For this review, take the finished solid that the model builds, in its own axes (mm). Coordinates: 2 decimals unless noted, no trailing zeros. Loops run counter-clockwise (first coordinate to the right, second up) from the corner with the lowest first, then second, coordinate; pieces in that order, holes last.
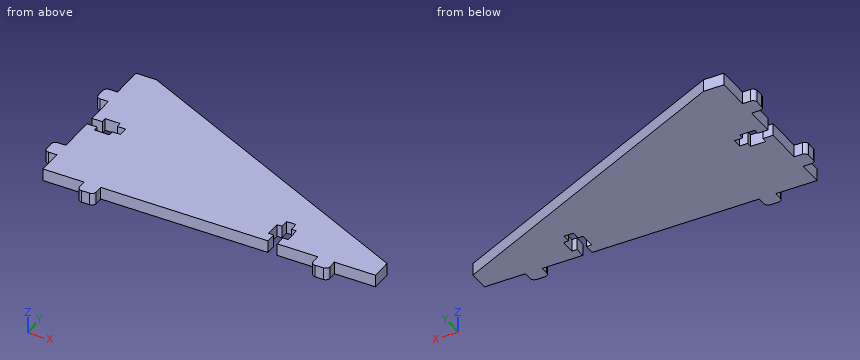
Autodesk Inventor part; units mm, degrees
ref_plane "YZ Plane" through (0, 0, 0) normal (1, 0, 0) x (0, 1, 0)
ref_plane "XZ Plane" through (0, 0, 0) normal (0, 1, 0) x (-1, 0, 0)
ref_plane "XY Plane" through (0, 0, 0) normal (0, 0, 1) x (1, 0, 0)
sketch "Sketch1" plane through (0, 0, 0) normal (0, 0, 1) x (1, 0, 0)
  line L0 (0, 81) -> (0, 0)
  line L1 (0, 0) -> (161.5, 0)
  line L2 (161.5, 0) -> (161.5, 10)
  line L3 (161.5, 10) -> (10, 81)
  line L4 (10, 81) -> (0, 81)
  dimension "d0" = 161.5
  dimension "d1" = 81
  dimension "d2" = 10
  dimension "d3" = 10
extrude "Extrusion1" add sketch "Sketch1" along normal blind 6
sketch "Sketch2" plane through (0, 0, 6) normal (0, 0, 1) x (1, 0, 0)
  line L0 (0, 81) -> (0, 0)
  line L1 (0, 0) -> (161.5, 0)
  line L2 (161.5, 0) -> (161.5, 10)
  line L3 (16.3, 42.75) -> (16.3, 38.25)
  line L4 (0, 38.25) -> (0, 42.75)
  line L5 (5, 45.25) -> (12.3, 45.25)
  line L6 (12.3, 35.75) -> (5, 35.75)
  line L7 (0, 42.75) -> (5, 42.75)
  line L8 (12.3, 42.75) -> (16.3, 42.75)
  line L9 (16.3, 38.25) -> (12.3, 38.25)
  line L10 (5, 38.25) -> (0, 38.25)
  line L11 (5, 35.75) -> (5, 38.25)
  line L12 (5, 42.75) -> (5, 45.25)
  line L13 (12.3, 45.25) -> (12.3, 42.75)
  line L14 (12.3, 38.25) -> (12.3, 35.75)
  line L15 (109.25, 16.3) -> (113.75, 16.3)
  line L16 (113.75, 0) -> (109.25, 0)
  line L17 (116.25, 12.3) -> (116.25, 5)
  line L18 (106.75, 5) -> (106.75, 12.3)
  line L19 (106.75, 12.3) -> (109.25, 12.3)
  line L20 (113.75, 12.3) -> (116.25, 12.3)
  line L21 (116.25, 5) -> (113.75, 5)
  line L22 (109.25, 5) -> (106.75, 5)
  line L23 (109.25, 0) -> (109.25, 5)
  line L24 (109.25, 12.3) -> (109.25, 16.3)
  line L25 (113.75, 16.3) -> (113.75, 12.3)
  line L26 (113.75, 5) -> (113.75, 0)
  point P0 (16.3, 40.5)
  point P1 (0, 40.5)
  point P2 (111.5, 16.3)
  dimension "d6" = 4.5
  dimension "d7" = 2.5
  dimension "d8" = 2.5
  dimension "d9" = 5
  dimension "d10" = 7.3
  dimension "d11" = 4
  dimension "d12" = 4.5
  dimension "d13" = 5
  dimension "d14" = 7.3
  dimension "d15" = 4
  dimension "d16" = 2.5
  dimension "d17" = 2.5
  dimension "d18" = 50
extrude "Extrusion2" cut sketch "Sketch2" against normal blind 6
sketch "Sketch3" plane through (0, 0, 6) normal (0, 0, 1) x (1, 0, 0)
  line L0 (0, 38.25) -> (0, 0)
  line L1 (0, 0) -> (109.25, 0)
  line L2 (113.75, 0) -> (161.5, 0)
  line L3 (10, 81) -> (0, 81)
  line L4 (0, 81) -> (0, 42.75)
  line L5 (0, 65) -> (-4, 65)
  line L6 (-6, 63) -> (-6, 59)
  line L7 (-4, 57) -> (0, 57)
  line L8 (0, 57) -> (0, 65)
  line L9 (0, 20) -> (-4, 20)
  line L10 (-6, 18) -> (-6, 14)
  line L11 (-4, 12) -> (0, 12)
  line L12 (0, 12) -> (0, 20)
  line L13 (20, 0) -> (28, 0)
  line L14 (28, 0) -> (28, -4)
  line L15 (26, -6) -> (22, -6)
  line L16 (20, -4) -> (20, 0)
  line L17 (133.5, 0) -> (141.5, 0)
  line L18 (141.5, 0) -> (141.5, -4)
  line L19 (139.5, -6) -> (135.5, -6)
  line L20 (133.5, -4) -> (133.5, 0)
  arc A0 (-4, 65) -> (-6, 63) centre (-4, 63) ccw
  arc A1 (-6, 59) -> (-4, 57) centre (-4, 59) ccw
  arc A2 (-4, 20) -> (-6, 18) centre (-4, 18) ccw
  arc A3 (-6, 14) -> (-4, 12) centre (-4, 14) ccw
  arc A4 (20, -4) -> (22, -6) centre (22, -4) ccw
  arc A5 (26, -6) -> (28, -4) centre (26, -4) ccw
  arc A6 (133.5, -4) -> (135.5, -6) centre (135.5, -4) ccw
  arc A7 (139.5, -6) -> (141.5, -4) centre (139.5, -4) ccw
  dimension "d21" = 2
  dimension "d22" = 8
  dimension "d23" = 8
  dimension "d24" = 8
  dimension "d25" = 8
  dimension "d26" = 6
  dimension "d27" = 6
  dimension "d28" = 12
  dimension "d29" = 16
  dimension "d30" = 20
  dimension "d31" = 20
extrude "Extrusion3" add sketch "Sketch3" against normal blind 6
properties part number "wiring_brace"
Q1. Consider section A-A (x = 67.5). State the section outline as (y, z) points.
Q2. Consider section B-B (y = 28). State the section outline as (x, z) points.
Q3. Wall thickness on probe 1 along X at (y, z) = (2.5, 5.15); probe 2 along X at (y, z) = (9, 3.35); probe 3 along Y at (x, z) = (153, 4.5): over which ranges is each line inside the solid? List them lowest first.
Q4. For pin 1 Ø1.5 at (y, z) = (27.5, 3.5) entering from -X; pin 2 Ø1.2 at (x, z) = (13.5, 3.5) entering from -Y; pin 3 Ø2 at (x, z) = (114.5, 1.5) entering from +Y, all flat-tipped, find the tip position at first contact; note any pin that passes through.
Model answer:
1. outline: (0, 0) - (54.05, 0) - (54.05, 6) - (0, 6) - close
2. outline: (0, 0) - (123.09, 0) - (123.09, 6) - (0, 6) - close
3. probe 1: x = 0 to 109.25, 113.75 to 161.5
3. probe 2: x = 0 to 106.75, 116.25 to 161.5
3. probe 3: y = 0 to 13.98
4. pin 1: stops at x = 0
4. pin 2: stops at y = 0
4. pin 3: stops at y = 32.5
